```python
from build123d import *

# Parameters (mm, degrees)
SKETCH2_R               = 15
SKETCH2_R_2             = 13
BOSS_EXTRUDE1_DEPTH     = 26.5
CUT_EXTRUDE1_REACH      = 35.945
CUT_EXTRUDE1_END_RADIUS = 15


with BuildPart() as part:
    # Sketch2 → Boss-Extrude1 (new, symmetric)
    with BuildSketch(Plane.XY):
        Circle(SKETCH2_R)
        Circle(SKETCH2_R_2, mode=Mode.SUBTRACT)
    extrude(amount=BOSS_EXTRUDE1_DEPTH, both=True)

    # Cut-Extrude1: up to this cylinder (the profile starts inside it)
    cut_extrude1_end = Plane(origin=(0, 0, 0), z_dir=(0, 0, -1)) * Cylinder(CUT_EXTRUDE1_END_RADIUS, 152.939652, mode=Mode.PRIVATE)
    # Sketch3 → Cut-Extrude1 (cut, up to the surface)
    with BuildSketch(Plane(origin=(0, 0, 0), x_dir=(0, 0, -1), z_dir=(1, 0, 0)), mode=Mode.PRIVATE) as cut_extrude1_sk1:
        with BuildLine():
            Line((-26.5, -3.75), (-24.5, -3.75))
            ThreePointArc((-24.5, -3.75), (-23.792893219, -3.457106781), (-23.5, -2.75))
            Line((-23.5, -2.75), (-23.5, 2.75))
            ThreePointArc((-23.5, 2.75), (-23.792893219, 3.457106781), (-24.5, 3.75))
            Line((-24.5, 3.75), (-26.5, 3.75))
            Line((-26.5, 3.75), (-26.5, -3.75))
        make_face()
    cut_extrude1_tool1 = extrude(cut_extrude1_sk1.sketch, amount=CUT_EXTRUDE1_REACH, mode=Mode.PRIVATE) & cut_extrude1_end
    add(cut_extrude1_tool1.solids().sort_by_distance((0, 0, 25.024826))[0], mode=Mode.SUBTRACT)
    # Sketch3 → Cut-Extrude1 (cut, up to the surface)
    with BuildSketch(Plane(origin=(0, 0, 0), x_dir=(0, 0, -1), z_dir=(1, 0, 0)), mode=Mode.PRIVATE) as cut_extrude1_sk2:
        with BuildLine():
            Line((26.5, -3.75), (24.5, -3.75))
            ThreePointArc((24.5, -3.75), (23.792893219, -3.457106781), (23.5, -2.75))
            Line((23.5, -2.75), (23.5, 2.75))
            ThreePointArc((23.5, 2.75), (23.792893219, 3.457106781), (24.5, 3.75))
            Line((24.5, 3.75), (26.5, 3.75))
            Line((26.5, 3.75), (26.5, -3.75))
        make_face()
    cut_extrude1_tool2 = extrude(cut_extrude1_sk2.sketch, amount=CUT_EXTRUDE1_REACH, mode=Mode.PRIVATE) & cut_extrude1_end
    add(cut_extrude1_tool2.solids().sort_by_distance((0, 0, -25.024826))[0], mode=Mode.SUBTRACT)


solid = part.part
```
Input: part model. Units: mm. Frame: model coordinates. A direction names the side the tool comes from. Give positions to 0.01 mm unless a question says otherwise; leave off trailing zeros. Order: outer loops, then holes, each group sorted by start corner. A loop starts at its lowest first (then second) coordinate and runs counter-clockwise, first axis right, second up. Notation, with made-up numbers: (0, -40) - (25, -40) arc R28 ccw to (25, -8) - close; hole circle Ø6 at (-28, 87). An arc over 180 degrees is marked (long way). Put each result on its own line as item: value.
Item 1: Section query B-B, the plane y = -12. Return loops of the section in (x, z), then the cut area to 3 significant figures.
Found:
outline: (-9, -26.5) - (-5, -26.5) - (-5, 26.5) - (-9, 26.5) - close; (5, -26.5) - (9, -26.5) - (9, 26.5) - (5, 26.5) - close
area: 424 mm^2
Item 2: Section query C-C, the plane z = -3.5. Return loops of the section in (x, y), then the cut area to 3 significant figures.
Found:
outline: circle Ø30 at (0, 0); hole circle Ø26 at (0, 0)
area: 176 mm^2
Item 3: Access query for faces 1 (the flat face through (13, -3.75, -26)), 2 (the flat face through (13, -3.75, 26)), 3 (the flat face through (-13.4, 0.1, 26.5)). Directions: +Z, -Z, +X, -X, +Y, -Y. A direction counts if a zero-diameter tool reaches every point of the face in a straight line with its end or side. Return the directions, or none.
Found:
face 1: -Z, +X
face 2: +Z, +X
face 3: +Z, +X, -X, +Y, -Y
Item 4: Ray query, L1, parallel to X at y = 0.5, z = -11.5; L2, parallel to X at y = -6, z = -8. Return the intervals inside material, ascending. Write a range as from..to.
Found:
L1: x = -14.99..-12.99, 12.99..14.99
L2: x = -13.75..-11.53, 11.53..13.75
Item 5: Section query A-A, the plane x = 0. Return loops of the section in (y, z), then the cut area to 3 significant figures.
Found:
outline: (-15, -26.5) - (-13, -26.5) - (-13, 26.5) - (-15, 26.5) - close; (13, -26.5) - (15, -26.5) - (15, 26.5) - (13, 26.5) - close
area: 212 mm^2
Item 6: Contact query for flat-ended pins moving along their axis: pin 1 (6 mm diameter, centred on x = 4.5, z = 8.5, fed in from -Y); pin 2 (1.6 mm diameter, centred on x = 13.5, z = -26, fed in from -Y); pin 3 (4 mm diameter, centred on x = 11, z = -3.5, fed in from -Y). Output: stop coordinate, or through.
Found:
pin 1: stops at y = -14.92
pin 2: stops at y = -7.98
pin 3: stops at y = -12
